```python
from build123d import *

# Parameters (mm, degrees)
SKETCH_1_R           = 30.073213795
SKETCH_1_R_2         = 19
EXTRUDE_1_DEPTH      = 44
EXTRUDE_2_DEPTH      = 12
EXTRUDE_3_DEPTH      = 16
EXTRUDE_3_DEPTH_BACK = 16
SKETCH_2_R           = 14
SKETCH_2_R_2         = 6


with BuildPart() as part:
    # Sketch 1 → Extrude 1 (new body)
    with BuildSketch(Plane(origin=(0, 0, 0), x_dir=(1, 0, 0), z_dir=(0, 1, 0))):
        with Locations(Location((0, 0.075325719, 0), (0, 0, 270))):
            Circle(SKETCH_1_R)
        with Locations(Location((0, 0.075325719, 0), (0, 0, 270))):
            Circle(SKETCH_1_R_2, mode=Mode.SUBTRACT)
    extrude(amount=EXTRUDE_1_DEPTH)

    # Sketch 1_3 → Extrude 2 (add)
    with BuildSketch(Plane(origin=(0, 0, 0), x_dir=(1, 0, 0), z_dir=(0, 1, 0))):
        with BuildLine():
            ThreePointArc((50, -8), (42, 0), (50, 8))
            Line((50, 8), (75, 8.150651437))
            ThreePointArc((75, 8.150651437), (73.70484886, 11.838399085), (70.413394867, 13.946296092))
            Line((70.413394867, 13.946296092), (7.08673549, 29.301621551))
            ThreePointArc((7.08673549, 29.301621551), (23.638095307, 18.666684955), (30.073213795, 0.075325719))
            ThreePointArc((30.073213795, 0.075325719), (23.633171917, -18.522291685), (7.071257605, -29.154718822))
            Line((7.071257605, -29.154718822), (70.4108085, -13.831776691))
            ThreePointArc((70.4108085, -13.831776691), (73.715127305, -11.710468232), (75, -8))
            Line((75, -8), (50, -8))
        make_face()
    extrude(amount=EXTRUDE_2_DEPTH)

    # Sketch 2 → Extrude 3 (add, two sides: drawn at the far end of the back side and taken through both)
    with BuildSketch(Plane.XY.offset(-EXTRUDE_3_DEPTH_BACK)):
        with Locations((-35.926786205, 14.387019523)):
            Circle(SKETCH_2_R)
        with Locations((-35.926786205, 14.387019523)):
            Circle(SKETCH_2_R_2, mode=Mode.SUBTRACT)
    extrude(amount=EXTRUDE_3_DEPTH + EXTRUDE_3_DEPTH_BACK)


solid = part.part
```
Could you check a few things on this model? Use its own coordinates, in mm. A direction names the side the tool comes from. Round coordinates to 2 decimals unless told otherwise and drop trailing zeros. Loops run counter-clockwise (first coordinate to the right, second up) from the corner with the lowest first, then second, coordinate; pieces in that order, holes last. Notation, with made-up numbers: (48.25, 47) - (94.25, 47) arc R9 ccw to (94.25, 57) - close; hole circle Ø3 at (46, 14). An arc over 180 degrees is marked (long way). Answer in a Markdown table with one row per item. Add a question column.
(1) For faces 1 (the face through (-38, 8, -16)), 2 (the face through (-38, 8, 16)), 3 (the face through (63, 6, 8)), 4 (the face through (-30.073, 14.369, -0.117)), which set-ups out of +Z, -Z, +X, -X, +Y, -Y let a thin tool reach every point of the face, with its end or its side?
(2) If we mould it in two halves opening along Y, with no side actions, what happens to faces 5 (the face through (73.739, 5.916, -11.795)), 6 (the face through (-41.92, 14.65, -0.22)), 7 (the face through (-20, 44, 0))? For each: pulls with the +Y half, pulls with the -Y half, needs draft (parallel to the pull), parting line crosses it, or undercut.
(3) I need wall thicknesses on line 1 along X through (y, z) = (17.5, -11); line 2 along X through (y, z) = (37, -9); line 3 along X through (y, z) = (16.5, 15.5). Which ranges of each line are inside material? Lowest first, please.
(4) I'm going to push flat-ended pins straight in: pin 1 (8 mm diameter, centred on x = 58, z = -20, fed in from +Y); pin 2 (13 mm diameter, centred on x = 63, y = 4, fed in from -Z); pin 3 (4 mm diameter, centred on y = 13, z = -10.5, fed in from +X); pin 4 (6 mm diameter, centred on x = 56, z = 5.5, fed in from -Y). Where does each tip first touch, or does it pass through?
(5) If we section it at B-B (z = 6): Please give me the cut outline in (x, y), plus the area to 3 significant figures.
(6) If we section it at C-C (y = 18): Please give me the cut outline in (x, z).
(7) If we section it at A-A (x = 0): Please give me the cut outline in (y, z), plus the area to 3 significant figures.
(8) If we section it at D-D (y = 10): Please give me the cut outline in (x, z), plus the area to 3 significant figures.
Model answer:
| question | item | result |
|---|---|---|
| 1 | face 1 | -Z, -X, +Y, -Y |
| 1 | face 2 | +Z, -X, +Y, -Y |
| 1 | face 3 | +X, +Y, -Y |
| 1 | face 4 | none |
| 2 | face 5 | needs draft |
| 2 | face 6 | undercut |
| 2 | face 7 | pulls with the +Y half |
| 3 | line 1 | x = -49.58 to -41.06, -30.8 to -15.55, 15.55 to 28.02 |
| 3 | line 2 | x = -28.72 to -16.77, 16.77 to 28.72 |
| 3 | line 3 | x = -49.77 to -41.54, -30.31 to -10.88, 10.88 to 25.73 |
| 4 | pin 1 | stops at y = 12 |
| 4 | pin 2 | stops at z = -17.32 |
| 4 | pin 3 | stops at x = 74.96 |
| 4 | pin 4 | stops at y = 0 |
| 5 | outline | (-29.45, 0) - (-18, 0) - (-18, 44) - (-29.45, 44) - (-29.45, 26.8) arc R14 ccw (long way) to (-29.45, 1.97) - close; (18, 0) - (44.71, 0) - (44.71, 12) - (29.45, 12) - (29.45, 44) - (18, 44) - close; hole circle Ø12 at (-35.93, 14.39) |
| 5 | area | 1,560 mm² |
| 6 | outline | (-49.45, -16) - (-40.72, -16) - (-40.72, 16) - (-49.45, 16) - close; (-31.14, -16) - (-25.51, -16) arc R30.07 ccw (long way) to (-25.42, 16) - (-31.14, 16) - close; hole circle Ø38 at (0, -0.08) |
| 7 | outline | (0, -30.15) - (44, -30.15) - (44, -19.08) - (0, -19.08) - close; (0, 18.92) - (44, 18.92) - (44, 30) - (0, 30) - close |
| 7 | area | 974 mm² |
| 8 | outline | (-49.22, -16) - (-40.02, -16) - (-40.02, 16) - (-49.22, 16) - close; (-31.83, -16) - (-25.51, -16) arc R30.07 ccw to (7.09, -29.3) - (70.41, -13.95) arc R6 ccw to (75, -8.15) - (50, -8) arc R8 cw to (50, 8) - (75, 8) arc R6 ccw to (70.41, 13.83) - (7.07, 29.15) arc R30.07 ccw to (-25.42, 16) - (-31.83, 16) - close; hole circle Ø38 at (0, -0.08) |
| 8 | area | 3,450 mm² |
